from build123d import *

# Parameters (mm, degrees)
F0_W     = 730
F0_H     = 440
F1_DEPTH = 30
F0_W_2   = 750
F0_H_2   = 460
F2_DEPTH = 450
F3_R     = 5


with BuildPart() as f1:
    # F0 (on Top) → F1 (new body)
    with BuildSketch(Plane.XY):
        with Locations((-1.938822, 0)):
            Rectangle(F0_W, F0_H)
    extrude(amount=F1_DEPTH)

    # F0 (on Top) → F2 (join)
    with BuildSketch(Plane.XY):
        with Locations((-1.938822, 0)):
            Rectangle(F0_W_2, F0_H_2)
        with Locations((-1.938822, 0)):
            Rectangle(F0_W, F0_H, mode=Mode.SUBTRACT)
    extrude(amount=F2_DEPTH)

    # F3
    f3_edges = [f1.edges().sort_by_distance(p)[0] for p in [
        (-376.938822, -230, 225),
        (373.061178, -230, 225),
        (373.061178, 230, 225),
        (-376.938822, 230, 225),
    ]]
    fillet(f3_edges, radius=F3_R)


solid = f1.part
Geometry check sheet. Reference: the model listing, model coordinates, mm. A direction names the side the tool comes from. Coordinates: 2 decimals unless noted, no trailing zeros. Order: outer loops, then holes, each group sorted by start corner. A loop starts at its lowest first (then second) coordinate and runs counter-clockwise, first axis right, second up. Notation, with made-up numbers: (47.5, -15.5) - (91.5, -15.5) arc R34 cw to (91.5, 20.5) - close; hole circle Ø5 at (71.25, -2.75). An arc over 180 degrees is marked (long way). Answer in a Markdown table with one row per item. Add a question column.
1) Cross-section at C-C, the plane y = -121. Record the cut outline in (x, z).
2) Material ranges on line 1 along Y through (x, z) = (10, 269); line 2 along X through (y, z) = (-153, 205); line 3 along Z through (x, y) = (317.5, -26), recorded low to high. Write a range as [from, to].
3) Cross-section at B-B, the plane x = 190. Record the cut outline in (y, z).
4) Release check for a two-part mould opening along Y. For faces 1 (the flat face through (363.061, -3, 237)), 2 (the flat face through (-7, -230, 222)), 3 (the flat face through (-366.939, -3, 237)), 4 (the flat face through (373.061, -3, 222)) record: +Y half, -Y half, draft (parallel to the pull), parting line (faces both ways), or undercut.
5) Gauge pin test, flat end, axial feed: P1, Ø10, axis at x = -288.5, y = 145.5, coming from the +Z side. Record the tip position at first contact, or that the pin passes through.
6) Set-up check for faces 5 (the flat face through (-376.939, -3, 222)), 6 (the flat face through (-7, -220, 237)): record each of +Z, -Z, +X, -X, +Y, -Y from which the full face is reachable in a straight line by a thin tool's end or side.
7) Cross-section at A-A, the plane z = 106.5. Record the cut outline in (x, y), then the cut area to 3 significant figures.
Check result:
| question | item | result |
|---|---|---|
| 1 | outline | (-376.94, 0) - (373.06, 0) - (373.06, 450) - (363.06, 450) - (363.06, 30) - (-366.94, 30) - (-366.94, 450) - (-376.94, 450) - close |
| 2 | line 1 | y = [-230, -220], [220, 230] |
| 2 | line 2 | x = [-376.94, -366.94], [363.06, 373.06] |
| 2 | line 3 | z = [0, 30] |
| 3 | outline | (-230, 0) - (230, 0) - (230, 450) - (220, 450) - (220, 30) - (-220, 30) - (-220, 450) - (-230, 450) - close |
| 4 | face 1 | undercut |
| 4 | face 2 | -Y half |
| 4 | face 3 | undercut |
| 4 | face 4 | draft |
| 5 | P1 | stops at z = 30 |
| 6 | face 5 | +Z, -Z, -X, +Y, -Y |
| 6 | face 6 | +Z |
| 7 | outline | (-376.94, -225) arc R5 ccw to (-371.94, -230) - (368.06, -230) arc R5 ccw to (373.06, -225) - (373.06, 225) arc R5 ccw to (368.06, 230) - (-371.94, 230) arc R5 ccw to (-376.94, 225) - close; hole (-366.94, -220) - (363.06, -220) - (363.06, 220) - (-366.94, 220) - close |
| 7 | area | 23,800 mm² |
